from build123d import *

# Parameters (mm, degrees)
SKETCH1_R           = 2
SKETCH1_R_2         = 1
SKETCH1_R_3         = 0.5
BOSS_EXTRUDE1_DEPTH = 1.6


with BuildPart() as part:
    # Sketch1 → Boss-Extrude1 (new body)
    with BuildSketch(Plane(origin=(0, 0, 0), x_dir=(0, 0, -1), z_dir=(1, 0, 0))):
        Polygon((0, 0), (0, 53), (120, 53), (129, 44.063430305), (129, 39.423430305), (61, 39.423430305), (61, -1.563926021), (51, -1.563926021), (51, -13.563926021), (16, -13.563926021), (16, 0), align=None)
        with Locations((13, 5)):
            Circle(SKETCH1_R, mode=Mode.SUBTRACT)
        with Locations((47, 5)):
            Circle(SKETCH1_R, mode=Mode.SUBTRACT)
        with Locations((47, 49)):
            Circle(SKETCH1_R, mode=Mode.SUBTRACT)
        with Locations((11, 50.35)):
            Circle(SKETCH1_R_2, mode=Mode.SUBTRACT)
        with Locations((21, 50.35)):
            Circle(SKETCH1_R_2, mode=Mode.SUBTRACT)
        with Locations((31, 50.35)):
            Circle(SKETCH1_R_2, mode=Mode.SUBTRACT)
        with Locations((123.861808856, 43.882900864)):
            Circle(SKETCH1_R_3, mode=Mode.SUBTRACT)
    extrude(amount=BOSS_EXTRUDE1_DEPTH)


solid = part.part
Read the model definition and answer for the solid it produces. Units are mm, in the model's axes. Give positions to 0.01 mm unless a question says otherwise; leave off trailing zeros. Write each loop counter-clockwise with the first axis right and the second up, starting at its lowest first coordinate (ties: lowest second). Pieces come first, ordered by that corner, then holes. Notation, with made-up numbers: (-29.75, 59) -> (20.25, 59) arc R9 ccw to (20.25, 74) -> close; hole circle Ø8 at (8.25, 81). An arc over 180 degrees is marked (long way). Answer as a JSON object with one key per item and string values. Group by question number.
1) Find section A-A (z = -47). Write down the section's boundary in (x, y), and give its area (3 significant figures).
2) Consider L1, parallel to Y at x = 0.55, z = -31; L2, parallel to Z at x = 1.05, y = 4; L3, parallel to Y at x = 0.9, z = -13. Determine where each line is inside the solid, lowest interval first. Write a range as from..to.
3) Find section B-B (y = 5). Write down the section's boundary in (x, z).
4) Each of these flat-tipped pins is pushed along its axis until it touches: P1, Ø1.8, axis at y = 50.35, z = -11, coming from the +X side; P2, Ø0.8, axis at x = 0.5, y = 13.5, coming from the -Z side; P3, Ø0.8, axis at x = 0.5, z = -54.5, coming from the -Y side. Where does it stop, or does it pass through?
5) The mould has two halves that part along Y. Classify faces 1 (the flat face through (1.6, 28, -51)), 2 (the flat face through (0.79, 48.59, -124.44)), 3 (the cylindrical face through (0.789, 47.226, -47.923)): +Y half, -Y half, draft (parallel to the pull), parting line (faces both ways), or undercut.
6) Find section D-D (z = -110). Write down the section's boundary in (x, y).
7) Find section C-C (x = 0.75). Write down the section's boundary in (y, z).
Values follow:
{
 "1": {"outline": "(0, -13.56) -> (1.6, -13.56) -> (1.6, 3) -> (0, 3) -> close; (0, 7) -> (1.6, 7) -> (1.6, 47) -> (0, 47) -> close; (0, 51) -> (1.6, 51) -> (1.6, 53) -> (0, 53) -> close", "area": "93.7 mm2"},
 "2": {"L1": "y = -13.56..49.35, 51.35..53", "L2": "z = -61..-48.73, -45.27..-14.73, -11.27..0", "L3": "y = 0..3, 7..53"},
 "3": {"outline": "(0, -61) -> (1.6, -61) -> (1.6, -49) -> (0, -49) -> close; (0, -45) -> (1.6, -45) -> (1.6, -15) -> (0, -15) -> close; (0, -11) -> (1.6, -11) -> (1.6, 0) -> (0, 0) -> close"},
 "4": {"P1": "passes through", "P2": "stops at z = -61", "P3": "stops at y = -1.56"},
 "5": {"face 1": "draft", "face 2": "+Y half", "face 3": "undercut"},
 "6": {"outline": "(0, 39.42) -> (1.6, 39.42) -> (1.6, 53) -> (0, 53) -> close"},
 "7": {"outline": "(-13.56, -51) -> (-1.56, -51) -> (-1.56, -61) -> (39.42, -61) -> (39.42, -129) -> (44.06, -129) -> (53, -120) -> (53, 0) -> (0, 0) -> (0, -16) -> (-13.56, -16) -> close; hole circle Ø4 at (5, -47); hole circle Ø4 at (5, -13); hole circle Ø1 at (43.88, -123.86); hole circle Ø4 at (49, -47); hole circle Ø2 at (50.35, -31); hole circle Ø2 at (50.35, -21); hole circle Ø2 at (50.35, -11)"}
}
